Could you check a few things on this model? Use its own coordinates, in mm. A direction names the side the tool comes from. Give positions to 0.01 mm unless a question says otherwise; leave off trailing zeros. Order: outer loops, then holes, each group sorted by start corner. A loop starts at its lowest first (then second) coordinate and runs counter-clockwise, first axis right, second up. Notation, with made-up numbers: (3.25, 15) -> (45.25, 15) arc R26 cw to (45.25, 44) -> close; hole circle Ø6 at (-0.75, -23.5). An arc over 180 degrees is marked (long way). Answer as CSV lines item,"result". Start each with the question number.
(1) We'd pull the mould along X, two halves only. Please class faces 3 (the face through (0, 5, -4)), 4 (the face through (19.1, 5.07, 9.14)), 5 (the face through (-0.3, 10, 2.4)): released by +X, released by -X, zero draft, split by the parting line, or undercut.
(2) I want a section at A-A (x = 13). Please give me the cut outline in (y, z), plus the area to 3 significant figures.
(3) I want a section at C-C (x = 3). Please give me the cut outline in (y, z).
(4) On a 3-axis mill with a long thin cutter (end or side, diameter ignored), from which of +Z, -Z, +X, -X, +Y, -Y can I reach the whole of each face in a straight line? I mean faces 1 (the face through (-19.14, 4.93, -9.1)), 2 (the face through (0, 8, 2)). Say none if no direction works.
(5) I want a section at D-D (z = -3.75). Please give me the cut outline in (x, y).
(6) I want a section at B-B (y = 1.5). Please give me the cut outline in (x, z).
(7) I need wall thicknesses on L1, parallel to X at y = 6.75, z = -1.5; L2, parallel to Z at x = 13, y = 7; L3, parallel to X at y = 9.25, z = -7.75. Which ranges of each line are inside material? Lowest first, please.
```python
from build123d import *

# Parameters (mm, degrees)
PAD_DEPTH    = 10
SKETCH001_R  = 2.1
POCKET_DEPTH = 10
FILLET_R     = 3
PAD001_DEPTH = 8


with BuildPart() as part:
    # Sketch → Pad (new body, symmetric)
    with BuildSketch(Plane.XY):
        with BuildLine():
            Line((-20, 10), (-20, 0))
            Line((-20, 0), (20, 0))
            Line((20, 0), (20, 10))
            Line((20, 10), (5, 10))
            ThreePointArc((-5, 10), (0, 5), (5, 10))
            Line((-20, 10), (-5, 10))
        make_face()
    extrude(amount=PAD_DEPTH, both=True)

    # Sketch001 → Pocket (cut)
    with BuildSketch(Plane.XZ):
        with Locations((-13, 0)):
            Circle(SKETCH001_R)
        with Locations((13, 0)):
            Circle(SKETCH001_R)
    extrude(amount=-POCKET_DEPTH, mode=Mode.SUBTRACT)

    # Fillet
    fillet_edges = [part.edges().sort_by_distance(p)[0] for p in [
        (-20, 5, -10),
        (20, 5, -10),
        (-20, 5, 10),
        (20, 5, 10),
    ]]
    fillet(fillet_edges, radius=FILLET_R)

    # Sketch002 → Pad001 (new body)
    with BuildSketch(Plane.XY.offset(10)):
        with BuildLine():
            ThreePointArc((-5, 10), (0, 5), (5, 10))
            Line((-5, 10), (5, 10))
        make_face()
    extrude(amount=-PAD001_DEPTH)


solid = part.part
```
Final values:
1,face 3,"undercut"
1,face 4,"released by +X"
1,face 5,"zero draft"
2,outline,"(0, -10) -> (10, -10) -> (10, -2.1) -> (0, -2.1) -> close; (0, 2.1) -> (10, 2.1) -> (10, 10) -> (0, 10) -> close"
2,area,"158 mm²"
3,outline,"(0, -10) -> (6, -10) -> (6, 2) -> (10, 2) -> (10, 10) -> (0, 10) -> close"
4,face 1,"-Z, -X, +Y, -Y"
4,face 2,"-Z, +Y"
5,outline,"(-20, 0) -> (20, 0) -> (20, 10) -> (5, 10) arc R5 cw to (-5, 10) -> (-20, 10) -> close"
6,outline,"(-20, -7) arc R3 ccw to (-17, -10) -> (17, -10) arc R3 ccw to (20, -7) -> (20, 7) arc R3 ccw to (17, 10) -> (-17, 10) arc R3 ccw to (-20, 7) -> close; hole circle Ø4.2 at (-13, 0); hole circle Ø4.2 at (13, 0)"
7,L1,"-20 to -14.47, -11.53 to -3.8, 3.8 to 11.53, 14.47 to 20"
7,L2,"-10 to -2.1, 2.1 to 10"
7,L3,"-19.9 to -4.94, 4.94 to 19.9"
